from build123d import *

# Parameters (mm, degrees)
SKETCH_1_W               = 24
SKETCH_1_H               = 28
EXTRUDE_2_DEPTH          = 4
SKETCH_1_5_R             = 0.5
EXTRUDE_4_DEPTH          = 2
EXTRUDE_5_DEPTH          = 25
EXTRUDE_5_DEPTH_BACK     = 15
SKETCH_1_6_W             = 4
SKETCH_1_6_H             = 28
SKETCH_1_6_W_2           = 24
SKETCH_1_6_H_2           = 4
SKETCH_1_6_W_3           = 16.5
CUT_EXTRUDE_1_DEPTH      = 54.490653389
CUT_EXTRUDE_1_DEPTH_BACK = 54.490653389
CUT_EXTRUDE_2_DEPTH      = 54.490653389
CUT_EXTRUDE_2_DEPTH_BACK = 54.490653389
CUT_EXTRUDE_4_DEPTH      = 54.490653389
CUT_EXTRUDE_4_DEPTH_BACK = 54.490653389


with BuildPart() as part:
    # Sketch 1 → Extrude 2 (new body)
    with BuildSketch(Plane(origin=(0, 0, 0), x_dir=(1, 0, 0), z_dir=(0, 1, 0))):
        with Locations((0, 2)):
            Rectangle(SKETCH_1_W, SKETCH_1_H)
        with BuildLine():
            Line((-1.989974874, -4.7), (-3.48245603, 10.15))
            ThreePointArc((-3.48245603, 10.15), (-0.175219713, 13.995611256), (3.5, 10.5))
            ThreePointArc((3.5, 10.5), (3.495611256, 10.324780287), (3.48245603, 10.15))
            Line((3.48245603, 10.15), (1.989974874, -4.7))
            ThreePointArc((1.989974874, -4.7), (0, -6.5), (-1.989974874, -4.7))
        make_face(mode=Mode.SUBTRACT)
    extrude(amount=EXTRUDE_2_DEPTH)

    # Sketch 1_5 → Extrude 4 (add)
    with BuildSketch(Plane(origin=(0, 0, 0), x_dir=(1, 0, 0), z_dir=(0, 1, 0))):
        with BuildLine():
            Line((1.989974874, -4.7), (3.48245603, 10.15))
            ThreePointArc((3.48245603, 10.15), (0, 14), (-3.48245603, 10.15))
            Line((-3.48245603, 10.15), (-1.989974874, -4.7))
            ThreePointArc((-1.989974874, -4.7), (0, -6.5), (1.989974874, -4.7))
        make_face()
        with Locations(Location((0, -2.5, 0), (0, 0, 270))):
            Circle(SKETCH_1_5_R, mode=Mode.SUBTRACT)
    extrude(amount=EXTRUDE_4_DEPTH)

    # Sketch 1_6 → Extrude 5 (add, two sides: drawn at the far end of the back side and taken through both)
    with BuildSketch(Plane(origin=(0, 0, 0), x_dir=(1, 0, 0), z_dir=(0, 1, 0)).offset(-EXTRUDE_5_DEPTH_BACK)):
        with Locations((-14, 2)):
            Rectangle(SKETCH_1_6_W, SKETCH_1_6_H)
        with Locations((14, 2)):
            Rectangle(SKETCH_1_6_W, SKETCH_1_6_H)
        with Locations((0, -14)):
            Rectangle(SKETCH_1_6_W_2, SKETCH_1_6_H_2)
        Polygon((-12, -12), (-16, -12), (-16, -12.312844089), (-16, -16), (-12, -16), align=None)
        Polygon((-16, -12.312844089), (-16, -12), (-32.5, -12), (-32.5, -16), (-16, -16), align=None)
        with Locations((14, -14)):
            Rectangle(SKETCH_1_6_W, SKETCH_1_6_H_2)
        with Locations((24.25, -14)):
            Rectangle(SKETCH_1_6_W_3, SKETCH_1_6_H_2)
    extrude(amount=EXTRUDE_5_DEPTH + EXTRUDE_5_DEPTH_BACK)

    # Sketch 5 → Cut-Extrude 1 (cut, two sides: drawn at the far end of the back side and taken through both)
    with BuildSketch(Plane.ZY.offset(-12).offset(-CUT_EXTRUDE_1_DEPTH_BACK)):
        Polygon((-16, 4), (12, 25), (-16, 25), align=None)
    extrude(amount=CUT_EXTRUDE_1_DEPTH + CUT_EXTRUDE_1_DEPTH_BACK, mode=Mode.SUBTRACT)

    # Sketch 6 → Cut-Extrude 2 (cut, two sides: drawn at the far end of the back side and taken through both)
    with BuildSketch(Plane.ZY.offset(-12).offset(-CUT_EXTRUDE_2_DEPTH_BACK)):
        Polygon((-16, 0), (12, -15), (-16, -15), align=None)
    extrude(amount=CUT_EXTRUDE_2_DEPTH + CUT_EXTRUDE_2_DEPTH_BACK, mode=Mode.SUBTRACT)

    # Sketch 8 → Cut-Extrude 4 (cut, two sides: drawn at the far end of the back side and taken through both)
    with BuildSketch(Plane.ZY.offset(-12).offset(-CUT_EXTRUDE_4_DEPTH_BACK)):
        Polygon((4.5, 4), (-16, 4), (0.673039493, 16.50477962), (12, 25), align=None)
    extrude(amount=CUT_EXTRUDE_4_DEPTH + CUT_EXTRUDE_4_DEPTH_BACK, mode=Mode.SUBTRACT)


solid = part.part
Input: part model. Units: mm. Frame: model coordinates. A direction names the side the tool comes from. Give positions to 0.01 mm unless a question says otherwise; leave off trailing zeros. Order: outer loops, then holes, each group sorted by start corner. A loop starts at its lowest first (then second) coordinate and runs counter-clockwise, first axis right, second up. Notation, with made-up numbers: (-32, 82) - (-27, 82) arc R12 cw to (-27, 90) - close; hole circle Ø7 at (-17, -21.75). An arc over 180 degrees is marked (long way). Write each question's results on one line, items separated by ' | '.
Item 1: Material intervals for line 1 along X through (y, z) = (0.4, 2.5); line 2 along X through (y, z) = (-10.5, 8.5); line 3 along Y through (x, z) = (-3.5, 7), sorted ascending.
A:
line 1: x = -16 to -0.5, 0.5 to 16 | line 2: x = -16 to -12, 12 to 16 | line 3: y = 0 to 4
Item 2: Section C-C (y = 9). Return loops of the section in (x, z).
A:
outline: (-32.5, 12) - (-16, 12) - (-16, 6.29) - (-12, 6.29) - (-12, 12) - (12, 12) - (12, 6.29) - (16, 6.29) - (16, 12) - (32.5, 12) - (32.5, 16) - (-32.5, 16) - close
Item 3: Section B-B (z = -3). Return loops of the section in (x, y), and give its area (3 significant figures).
A:
outline: (-16, -6.96) - (-12, -6.96) - (-12, 0) - (12, 0) - (12, -6.96) - (16, -6.96) - (16, 4) - (2.76, 4) - (2.76, 2) - (-2.76, 2) - (-2.76, 4) - (-16, 4) - close | area: 173 mm^2
Item 4: Section D-D (x = -5.5). Return loops of the section in (y, z).
A:
outline: (-15, 12) - (0, 12) - (0, -16) - (4, -16) - (4, 12) - (25, 12) - (25, 16) - (-15, 16) - close
Item 5: Draft query along Z for faces 5 (the flat face through (0, 14, 12)), 6 (the flat face through (-12, -4, 4)), 7 (the flat face through (0, 5, 16)), 8 (the flat face through (-2.726, 2.986, -2.621)). Return one class per face: released by +Z, released by -Z, zero draft, split by the parting line, or undercut.
A:
face 5: released by -Z | face 6: zero draft | face 7: released by +Z | face 8: undercut
Item 6: Contact query for flat-ended pins moving along their axis: pin 1 Ø1 at (x, z) = (13.5, 3.5) entering from +Y; pin 2 Ø3 at (y, z) = (20.5, 11.5) entering from -X; pin 3 Ø13 at (x, y) = (27, 2.5) entering from -Z; pin 4 Ø7.5 at (y, z) = (-4, 1) entering from -X. Output: stop coordinate, or through.
A:
pin 1: stops at y = 4 | pin 2: stops at x = -32.5 | pin 3: stops at z = 12 | pin 4: stops at x = -16
Item 7: Access query for faces 1 (the flat face through (12, 12, 9)), 2 (the flat face through (16, 0, 2)), 3 (the flat face through (-24, 5, 12)), 4 (the flat face through (0, 0, -2)). Directions: +Z, -Z, +X, -X, +Y, -Y. A direction counts if a zero-diameter tool reaches every point of the face in a straight line with its end or side. Return the directions, or none.
A:
face 1: -Z, +Y | face 2: -Z, +X, +Y, -Y | face 3: -Z, -X, +Y, -Y | face 4: -Z, -Y
Item 8: Section A-A (x = -14.5). Return loops of the section in (y, z).
A:
outline: (-15, 12) - (0, -16) - (4, -16) - (4, 4.5) - (25, 12) - (25, 16) - (-15, 16) - close
